Here's the drawing with two shaded views (mm, measured from the low corner). I have some questions. Coordinates: 2 decimals unless noted, no trailing zeros. Loops run counter-clockwise (first coordinate to the right, second up) from the corner with the lowest first, then second, coordinate; pieces in that order, holes last. Notation, with made-up numbers: M 63.25,54 L 113.25,54 A28 cw 113.25,90 Z; hole C 44,-27.75 d1. An arc over 180 degrees is marked long. Use one line per item in the form item = value. Start each with the question number.
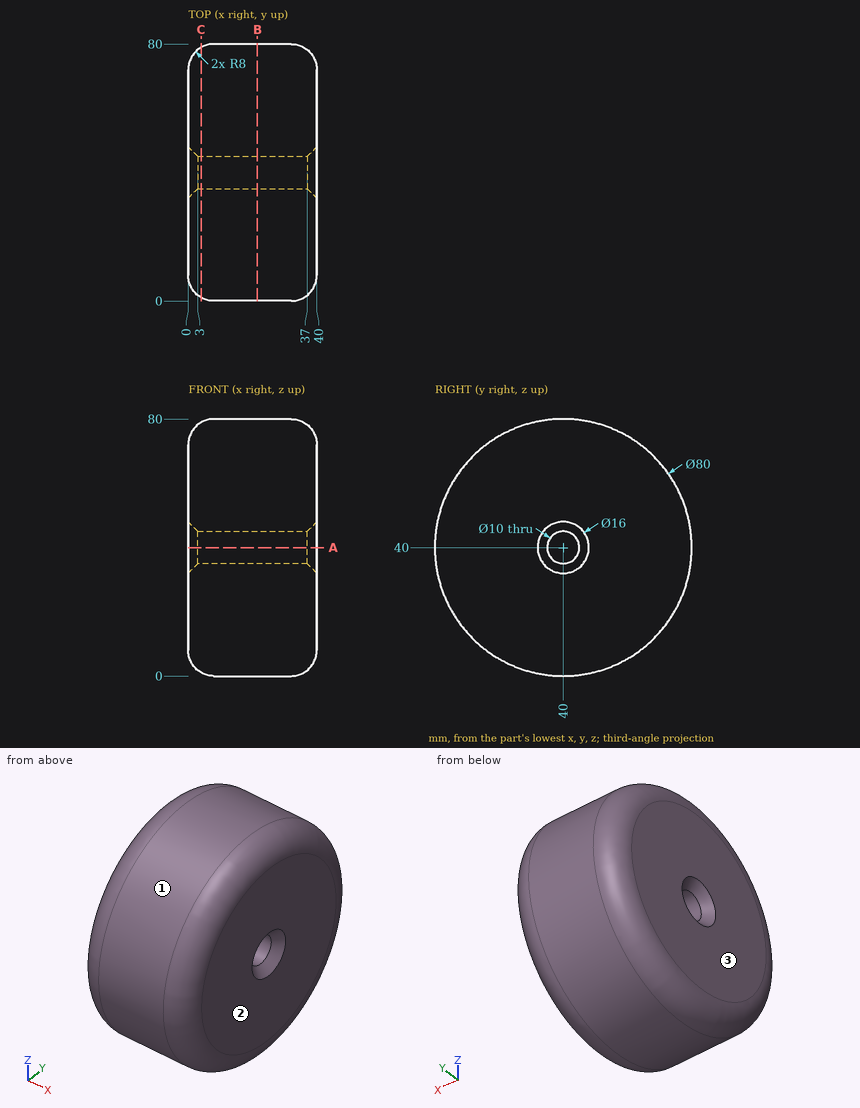
Item 1: I want a section at A-A (z = 40). Write out the boundary of the cut face in (x, y).
Item 2: I want a section at C-C (x = 4). Write out the boundary of the cut face in (y, z), plus the area to 3 significant figures.
Item 3: Please list where these lines run through material, in increasing order: line 1 along Y through (x, z) = (30, 40); line 2 along Y through (x, z) = (3.5, 43.5); line 3 along Z through (x, y) = (23.5, 54).
Item 4: I want a section at B-B (x = 21.5). Write out the boundary of the cut face in (y, z), plus the area to 3 significant figures.
Item 5: Thinking about a two-plate mould opening in X: for the marked faces 1, 2 and 3, which applies, pulls with the +X half, pulls with the -X half, needs draft (parallel to the pull), parting line crosses it, or undercut?
Item 6: I'm going to push flat-ended pins straight in: P1, Ø2, axis at x = 18, z = 19.5, coming from the -Y side; P2, Ø10, axis at y = 15.5, z = 13, coming from the -X side; P3, Ø8, axis at y = 14.5, z = 9.5, coming from the -X side; P4, Ø1, axis at x = 5.5, z = 42, coming from the +Y side. Where does each tip first touch, or does it pass through?
Worked answers:
q1.outline = M 0,8 A8 ccw 8,0 L 32,0 A8 ccw 40,8 L 40,32 L 37,35 L 3,35 L 0,32 Z; M 0,48 L 3,45 L 37,45 L 40,48 L 40,72 A8 ccw 32,80 L 8,80 A8 ccw 0,72 Z
q2.outline = C 40,40 d77.86; hole C 40,40 d10
q2.area = 4,680 mm²
q3.line_1 = 0 to 35, 45 to 80
q3.line_2 = 1.54 to 36.43, 43.57 to 78.46
q3.line_3 = 2.53 to 77.47
q4.outline = C 40,40 d80; hole C 40,40 d10
q4.area = 4,950 mm²
q5.face_1 = needs draft
q5.face_2 = pulls with the +X half
q5.face_3 = pulls with the -X half
q6.P1 = 5.08
q6.P2 = 0
q6.P3 = 0.94
q6.P4 = 79.7
